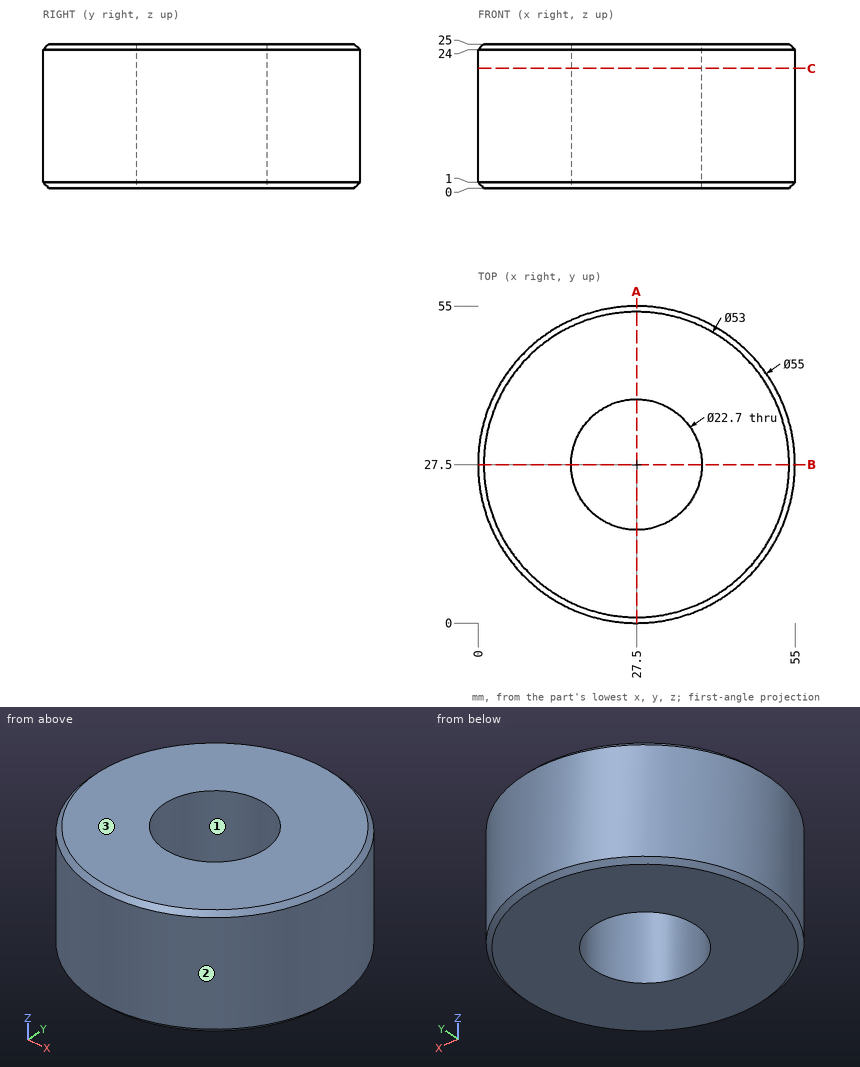
Could you check a few things on this drawing? It's one solid part, dimensions in mm from its lowest x, y, z. Coordinates: 2 decimals unless noted, no trailing zeros. Loops run counter-clockwise (first coordinate to the right, second up) from the corner with the lowest first, then second, coordinate; pieces in that order, holes last.
1. Imagine slicing it at A-A (x = 27.5). Please give me the cut outline in (y, z), and give its area (4 significant figures).
2. I need wall thicknesses on L1, parallel to Y at x = 27.5, z = 8.75; L2, parallel to Y at x = 37, z = 17; L3, parallel to X at y = 18.5, z = 8.75. Which ranges of each line are inside material? Lowest first, please.
3. We'd pull the mould along Y, two halves only. Please class the marked faces 1, 2 and 3: released by +Y, released by -Y, zero draft, split by the parting line, or undercut.
4. For P1, Ø2, axis at y = 33.5, z = 8.5, coming from the +X side; P2, Ø1, axis at x = 21, z = 12.5, coming from the -Y side; P3, Ø5, axis at x = 30, z = 9, coming from the +Y side, each with a flat end and sliding along its axis, tell me the tip position at first contact or that it passes through.
5. Imagine slicing it at C-C (z = 20.75). Please give me the cut outline in (x, y), and give its area (3 significant figures).
Computed values:
1. outline: (0, 1) - (1, 0) - (16.15, 0) - (16.15, 25) - (1, 25) - (0, 24) - close; (38.85, 0) - (54, 0) - (55, 1) - (55, 24) - (54, 25) - (38.85, 25) - close
1. area: 805.5 mm2
2. L1: y = 0 to 16.15, 38.85 to 55
2. L2: y = 1.69 to 21.29, 33.71 to 53.31
2. L3: x = 1.51 to 20.58, 34.42 to 53.49
3. face 1: undercut
3. face 2: split by the parting line
3. face 3: zero draft
4. P1: stops at x = 54.54
4. P2: stops at y = 0.66
4. P3: stops at y = 55
5. outline: circle Ø55 at (27.5, 27.5); hole circle Ø22.7 at (27.5, 27.5)
5. area: 1,970 mm2
